Can you work these out from the model? Positions are in its coordinate system, mm. Give positions to 0.01 mm unless a question says otherwise; leave off trailing zeros. Loops run counter-clockwise (first coordinate to the right, second up) from the corner with the lowest first, then second, coordinate; pieces in that order, holes last. Notation, with made-up numbers: (-29.5, -4.75) - (19.5, -4.75) arc R27 cw to (19.5, 16.25) - close; hole circle Ø1 at (14.25, 53). An arc over 180 degrees is marked (long way). Answer as a JSON object with one key per item and string values.
```python
from build123d import *

# Parameters (mm, degrees)
SKETCH1_W             = 146.05
SKETCH1_H             = 191.77
BOSS_EXTRUDE1_DEPTH   = 1.1938
F_8_CLEARANCE_HOLE1_D = 4.4958


with BuildPart() as part:
    # Sketch1 → Boss-Extrude1 (new body, symmetric)
    with BuildSketch(Plane.XY):
        Rectangle(SKETCH1_W, SKETCH1_H)
    extrude(amount=BOSS_EXTRUDE1_DEPTH, both=True)

    # #8 Clearance Hole1 (through all)
    with Locations(Plane(origin=(68.5165, 69.85, 1.1938), x_dir=(1, 0, 0), z_dir=(0, 0, 1))):
        with Locations((0, 0), (-137.033, 0), (-137.033, -139.7), (0, -139.7)):
            Hole(F_8_CLEARANCE_HOLE1_D / 2)


solid = part.part
```
1) I'm going to push a flat-ended pin straight in: P1, Ø4, axis at x = -68.52, y = 69.85, coming from the +Z side. Where does the tip first touch, or does it pass through?
Check sheet entries:
{"P1": "through"}
2) If we mould it in two halves opening along Y, with no side actions, what happens to faces 1 (the cylindrical face through (66.372, -69.175, -0.017)), 2 (the cylindrical face through (66.372, 70.525, -0.017)), 3 (the flat face through (-1, 1, -1.194))? For each: released by +Y, released by -Y, zero draft, split by the parting line, or undercut.
Check sheet entries:
{"face 1": "undercut", "face 2": "undercut", "face 3": "zero draft"}
3) Imagine slicing it at A-A on y = -69.85. Write out the boundary of the cut face in (x, z) (3 decimals).
Check sheet entries:
{"outline": "(-73.025, -1.194) - (-70.764, -1.194) - (-70.764, 1.194) - (-73.025, 1.194) - close; (-66.269, -1.194) - (66.269, -1.194) - (66.269, 1.194) - (-66.269, 1.194) - close; (70.764, -1.194) - (73.025, -1.194) - (73.025, 1.194) - (70.764, 1.194) - close"}
4) I need wall thicknesses on L1, parallel to X at y = -71, z = -0.05 (3 decimals). Which ranges of the line are inside material? Lowest first, please.
Check sheet entries:
{"L1": "-73.025 to -70.448, -66.585 to 66.585, 70.448 to 73.025"}
